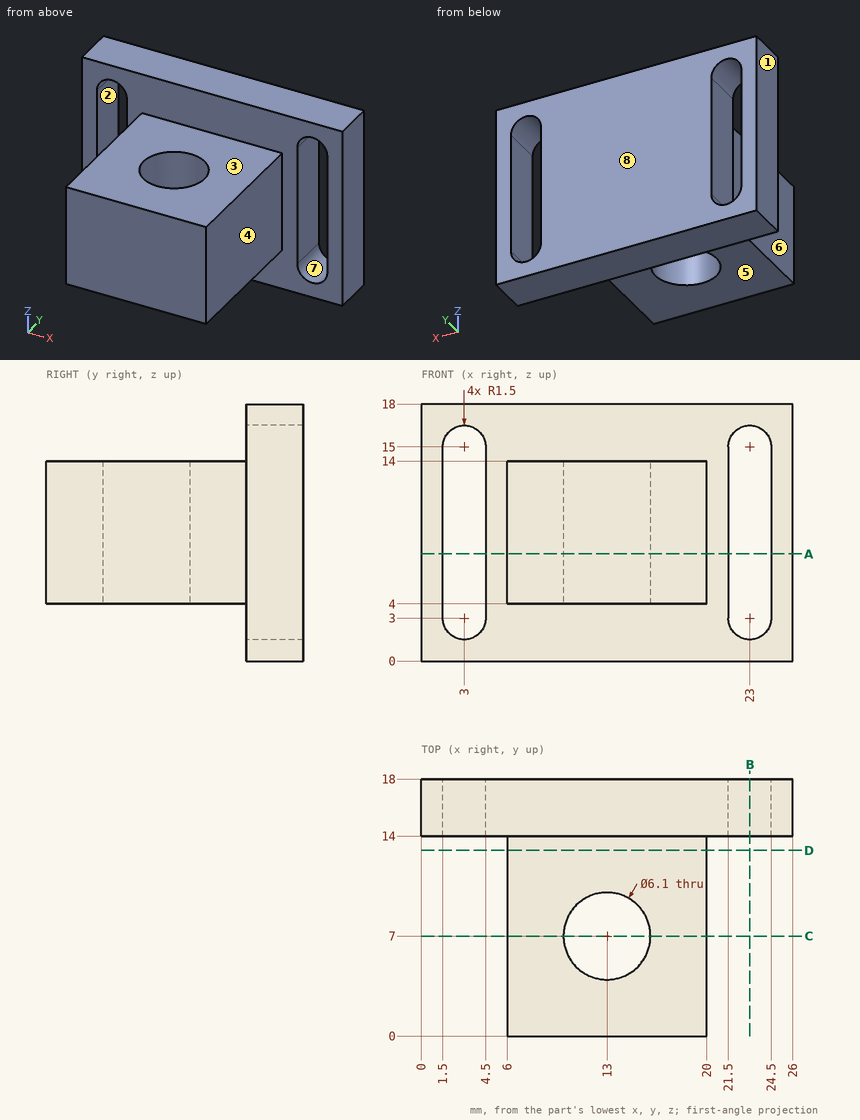
Study the drawing (mm; zero at the part's minimum x, y, z) and answer. A direction names the side the tool comes from. Round coordinates to 2 decimals unless told otherwise and drop trailing zeros. Write each loop counter-clockwise with the first axis right and the second up, starting at its lowest first coordinate (ties: lowest second). Pieces come first, ordered by that corner, then holes.
1) A cutting plane is placed at B-B on x = 23. Determine the outline of the cut face in (y, z).
2) Flat-ended cylindrical pins translate along their axes: P1, Ø8, axis at y = 8.5, z = 5, coming from the +X side; P2, Ø8, axis at x = 13, y = 7, coming from the -Z side; P3, Ø5, axis at x = 12.5, y = 8, coming from the +Z side. Find the tip coordinate at first contact, or state that the pin passes through.
3) Determine the mould class of the marked faces 1, 2 and 3 for opening direction Z: pulls with the +Z half, pulls with the -Z half, needs draft (parallel to the pull), parting line crosses it, or undercut.
4) A cutting plane is placed at A-A on z = 7.5. Determine the outline of the cut face in (x, y).
5) Consider probe 1 along X at (y, z) = (17, 7.5); probe 2 along Y at (x, z) = (13, 8.75); probe 3 along Y at (x, z) = (20.25, 14.5). Determine where each line is inside the solid, lowest interval first.
6) Which of the six approach directions +Z, -Z, +X, -X, +Y, -Y give full straight-line access (tool end or side, diameter ignored) to the marked faces 4, 5, 6, 7 and 8?
7) A cutting plane is placed at C-C on y = 7. Determine the outline of the cut face in (x, z).
8) A cutting plane is placed at D-D on y = 13. Determine the outline of the cut face in (x, z).
Entries:
1. outline: (14, 0) - (18, 0) - (18, 1.5) - (14, 1.5) - close; (14, 16.5) - (18, 16.5) - (18, 18) - (14, 18) - close
2. P1: stops at x = 20
2. P2: stops at z = 4
2. P3: stops at z = 14
3. face 1: needs draft
3. face 2: undercut
3. face 3: pulls with the +Z half
4. outline: (0, 14) - (1.5, 14) - (1.5, 18) - (0, 18) - close; (4.5, 14) - (6, 14) - (6, 0) - (20, 0) - (20, 14) - (21.5, 14) - (21.5, 18) - (4.5, 18) - close; (24.5, 14) - (26, 14) - (26, 18) - (24.5, 18) - close; hole circle Ø6.1 at (13, 7)
5. probe 1: x = 0 to 1.5, 4.5 to 21.5, 24.5 to 26
5. probe 2: y = 0 to 3.95, 10.05 to 18
5. probe 3: y = 14 to 18
6. face 4: +Z, -Z, +X, -Y
6. face 5: -Z, +X, -X, -Y
6. face 6: +Z, -Z, -X, -Y
6. face 7: +Y, -Y
6. face 8: +Z, -Z, +X, -X, +Y
7. outline: (6, 4) - (9.95, 4) - (9.95, 14) - (6, 14) - close; (16.05, 4) - (20, 4) - (20, 14) - (16.05, 14) - close
8. outline: (6, 4) - (20, 4) - (20, 14) - (6, 14) - close
